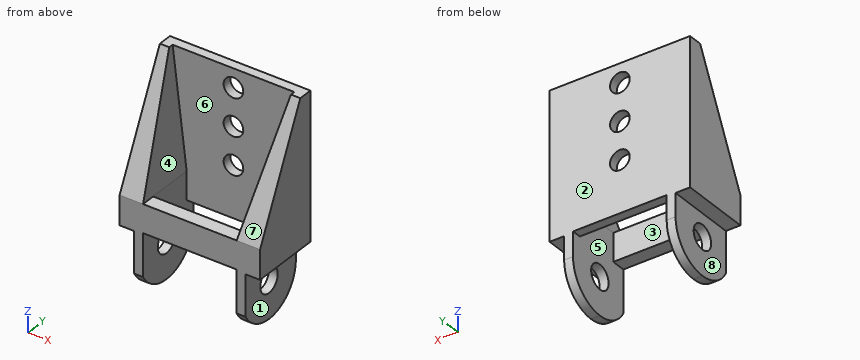
```python
from build123d import *

# Parameters (mm, degrees)
SKETCH_1_W               = 30
SKETCH_1_H               = 15
EXTRUDE_1_DEPTH          = 18
CUT_EXTRUDE_1_REACH      = 28.843
SKETCH_2_W               = 20
SKETCH_2_H               = 10
CUT_EXTRUDE_2_REACH      = 29.668
SKETCH_3_W               = 20
SKETCH_3_H               = 12
EXTRUDE_4_DEPTH          = 20
SKETCH_10_R              = 2.6
CUT_EXTRUDE_8_DEPTH      = 35.965796737
CUT_EXTRUDE_9_DEPTH      = 35.965796737
CUT_EXTRUDE_9_DEPTH_BACK = 35.965796737
SKETCH_12_W              = 1.696031958
SKETCH_12_H              = 15
SKETCH_17_W              = 3.1
SKETCH_17_H              = 15
EXTRUDE_8_DEPTH          = 0.27
EXTRUDE_9_DEPTH          = 13
CHAMFER_1_SIZE           = 25
CHAMFER_1_SIZE2          = 12
SKETCH_19_R              = 2.1
CUT_EXTRUDE_10_DEPTH     = 13
CHAMFER_2_SIZE           = 25
CHAMFER_2_SIZE_2         = 3


with BuildPart() as part:
    # 草圖1 → 填料-伸長1 (new body)
    with BuildSketch(Plane.XY):
        with Locations((2.249045701, -2.44972067)):
            Rectangle(SKETCH_1_W, SKETCH_1_H)
    extrude(amount=EXTRUDE_1_DEPTH)

    # 草圖2 → 除料-伸長1 (cut, up to next)
    with BuildSketch(Plane.XY.offset(18), mode=Mode.PRIVATE) as cut_extrude_1_sk1:
        with Locations((2.249045701, -1.94972067)):
            Rectangle(SKETCH_2_W, SKETCH_2_H)
    cut_extrude_1_tool1 = extrude(cut_extrude_1_sk1.sketch, amount=-CUT_EXTRUDE_1_REACH, mode=Mode.PRIVATE) & part.part
    add(cut_extrude_1_tool1.solids().sort_by_distance((2.249046, -1.949721, 18))[0], mode=Mode.SUBTRACT)

    # 草圖3 → 除料-伸長2 (cut, up to next)
    with BuildSketch(Plane(origin=(0, -6.94972067, 0), x_dir=(1, 0, 0), z_dir=(0, 1, 0)), mode=Mode.PRIVATE) as cut_extrude_2_sk1:
        with Locations((2.249045701, -12)):
            Rectangle(SKETCH_3_W, SKETCH_3_H)
    cut_extrude_2_tool1 = extrude(cut_extrude_2_sk1.sketch, amount=-CUT_EXTRUDE_2_REACH, mode=Mode.PRIVATE) & part.part
    add(cut_extrude_2_tool1.solids().sort_by_distance((2.249046, -6.949721, 12))[0], mode=Mode.SUBTRACT)

    # 草圖9 → 填料-伸長4 (add)
    with BuildSketch(Plane(origin=(0, 0, 0), x_dir=(-1, 0, 0), z_dir=(0, 0, -1))):
        Polygon((9.650954299, 5.05027933), (7.750954299, 5.05027933), (7.750954299, 3.05027933), (7.750954299, -6.94972067), (7.750954299, -9.94972067), (9.650954299, -9.94972067), align=None)
        Polygon((-12.249045701, 3.05027933), (-12.249045701, 5.05027933), (-14.149045701, 5.05027933), (-14.149045701, -9.94972067), (-12.249045701, -9.94972067), (-12.249045701, -6.94972067), align=None)
    extrude(amount=EXTRUDE_4_DEPTH)

    # 草圖10 → 除料-伸長8 (cut, through all)
    with BuildSketch(Plane(origin=(14.149045701, 0, 0), x_dir=(0, 0, -1), z_dir=(1, 0, 0))):
        with Locations((5.2, -2.94972067)):
            Circle(SKETCH_10_R)
    extrude(amount=-CUT_EXTRUDE_8_DEPTH, mode=Mode.SUBTRACT)

    # 草圖12 → 除料-伸長9 (cut, two sides: drawn at the far end of the back side and taken through both)
    with BuildSketch(Plane(origin=(14.149045701, 0, 0), x_dir=(0, 0, -1), z_dir=(1, 0, 0)).offset(-CUT_EXTRUDE_9_DEPTH_BACK)):
        with BuildLine():
            Line((18.303968042, 5.05027933), (5.2, 5.05027933))
            ThreePointArc((5.2, 5.05027933), (10.856854249, 2.707133579), (13.2, -2.94972067))
            ThreePointArc((13.2, -2.94972067), (12.091439137, -7.012732683), (9.072983346, -9.94972067))
            Line((9.072983346, -9.94972067), (18.303968042, -9.94972067))
            Line((18.303968042, -9.94972067), (18.303968042, 5.05027933))
        make_face()
        with Locations((19.151984021, -2.44972067)):
            Rectangle(SKETCH_12_W, SKETCH_12_H)
    extrude(amount=CUT_EXTRUDE_9_DEPTH + CUT_EXTRUDE_9_DEPTH_BACK, mode=Mode.SUBTRACT)

    # 草圖17 → 填料-伸長8 (add)
    with BuildSketch(Plane(origin=(0, 0, 0), x_dir=(-1, 0, 0), z_dir=(0, 0, -1))):
        with Locations((-15.699045701, -2.44972067)):
            Rectangle(SKETCH_17_W, SKETCH_17_H)
        with Locations((11.200954299, -2.44972067)):
            Rectangle(SKETCH_17_W, SKETCH_17_H)
    extrude(amount=EXTRUDE_8_DEPTH)

    # 草圖18 → 填料-伸長9 (add)
    with BuildSketch(Plane.XY.offset(18)):
        Polygon((-12.750954299, 5.05027933), (-12.750954299, -9.94972067), (-7.750954299, -9.94972067), (-7.750954299, 3.05027933), (12.249045701, 3.05027933), (12.249045701, -9.94972067), (17.249045701, -9.94972067), (17.249045701, 5.05027933), align=None)
    extrude(amount=EXTRUDE_9_DEPTH)

    # 導角1
    chamfer_1_edges = [part.edges().sort_by_distance(p)[0] for p in [
        (14.749045701, -9.94972067, 31),
        (-10.250954299, -9.94972067, 31),
    ]]
    chamfer_1_side = [part.faces().sort_by_distance(p)[0] for p in [
        (13.648461643, -9.94972067, -4.671491673),
    ]]
    chamfer(chamfer_1_edges, length=CHAMFER_1_SIZE, length2=CHAMFER_1_SIZE2, reference=chamfer_1_side[0])

    # 草圖19 → 除料-伸長10 (cut)
    with BuildSketch(Plane(origin=(0, 3.05027933, 0), x_dir=(-1, 0, 0), z_dir=(0, -1, 0))):
        with Locations(Location((-2.249045701, -27, 0), (0, 0, 90))):
            Circle(SKETCH_19_R)
        with Locations(Location((-2.249045701, -19, 0), (0, 0, 90))):
            Circle(SKETCH_19_R)
        with Locations(Location((-2.249045701, -11, 0), (0, 0, 90))):
            Circle(SKETCH_19_R)
    extrude(amount=-CUT_EXTRUDE_10_DEPTH, mode=Mode.SUBTRACT)

    # 導角2
    # the kernel refuses this chamfer: 25, 3 mm, written as the material it takes off along each edge
    with BuildSketch(Plane(origin=(12.249045701, 3.05027933, 31), x_dir=(-0.004583716135178889, 0, -0.9999894947180156), z_dir=(0, -1, 0)), Plane(origin=(-7.750954299, -62.93259543, 31), x_dir=(0.004583716135178923, 0, -0.9999894947180156), z_dir=(0, 1, 0))) as chamfer_2_piece_1:
        Polygon((CHAMFER_2_SIZE * 0.999989494718, CHAMFER_2_SIZE * 0.00458371613518), (-CHAMFER_2_SIZE_2 * 0.00458371613518, CHAMFER_2_SIZE_2 * 0.999989494718), (0, 0), align=None)
    extrude(amount=65.98287476, mode=Mode.SUBTRACT)


solid = part.part
```
CAD build for the part. Positions are in the model's coordinates, mm. Face numbers are marked on the shaded views. A direction names the side the tool comes from. Round coordinates to 2 decimals unless told otherwise and drop trailing zeros. Order: outer loops, then holes, each group sorted by start corner. A loop starts at its lowest first (then second) coordinate and runs counter-clockwise, first axis right, second up. Notation, with made-up numbers: (51, 55) - (60, 55) arc R29 cw to (60, 79) - close; hole circle Ø6 at (-14, 22). An arc over 180 degrees is marked (long way). Answer in a Markdown table with one row per item. Add a question column.
(1) Probe L1, parallel to X at y = -2, z = 3; L2, parallel to Y at x = 8.75, z = 4; L3, parallel to X at y = 3.85, z = 27. List the from-to ranges inside material, lowest first. Write a range as [from, to].
(2) Drop flat-ended pins along their axis: pin 1 Ø2.5 at (x, y) = (-11.5, -6) entering from -Z; pin 2 Ø8 at (x, y) = (10, -8) entering from -Z; pin 3 Ø8.5 at (y, z) = (-2.95, -5.2) entering from +X. Give the stop position or say it passes through.
(3) Band-saw the part on B-B on z = -10. List the corners of the cut face in (x, y).
(4) Band-saw the part on A-A on x = -6.75. List the corners of the cut face in (y, z), and give its area (3 significant figures).
(5) Mould opens along Y. For the marked faces 6, 7 and 8 say: +Y half, -Y half, draft (parallel to the pull), parting line (faces both ways), or undercut.
(6) Band-saw the part on D-D on x = 3. List the corners of the cut face in (y, z), and give its area (3 significant figures).
(7) 3-axis set-ups, long thin cutter, end or side, ignore diameter. For the marked faces 1, 2, 3, 4 and 5: which of +Z, -Z, +X, -X, +Y, -Y reach the whole face in a straight line?
(8) Band-saw the part on C-C on y = 0.75. List the corners of the cut face in (x, z).
Data:
| question | item | result |
|---|---|---|
| 1 | L1 | x = [-12.75, -7.75], [12.25, 17.25] |
| 1 | L2 | y = [-9.95, -6.95], [3.05, 5.05] |
| 1 | L3 | x = [-12.75, 0.15], [4.35, 17.25] |
| 2 | pin 1 | stops at z = -0.27 |
| 2 | pin 2 | stops at z = -13.01 |
| 2 | pin 3 | stops at x = 14.15 |
| 3 | outline | (-9.65, -9.35) - (-7.75, -9.35) - (-7.75, 3.45) - (-9.65, 3.45) - close; (12.25, -9.35) - (14.15, -9.35) - (14.15, 3.45) - (12.25, 3.45) - close |
| 4 | outline | (-9.95, 0) - (-6.95, 0) - (-6.95, 6) - (-9.95, 6) - close; (3.05, 0) - (5.05, 0) - (5.05, 31) - (3.05, 31) - close |
| 4 | area | 80.0 mm^2 |
| 5 | face 6 | undercut |
| 5 | face 7 | -Y half |
| 5 | face 8 | draft |
| 6 | outline | (-9.95, 0) - (-6.95, 0) - (-6.95, 6) - (-9.95, 6) - close; (3.05, 0) - (5.05, 0) - (5.05, 9.04) - (3.05, 9.04) - close; (3.05, 12.96) - (5.05, 12.96) - (5.05, 17.04) - (3.05, 17.04) - close; (3.05, 20.96) - (5.05, 20.96) - (5.05, 25.04) - (3.05, 25.04) - close; (3.05, 28.96) - (5.05, 28.96) - (5.05, 31) - (3.05, 31) - close |
| 6 | area | 56.5 mm^2 |
| 7 | face 1 | -Z, +X, +Y, -Y |
| 7 | face 2 | +Z, -Z, +X, -X, +Y |
| 7 | face 3 | +Z, -Z |
| 7 | face 4 | +Z, -Y |
| 7 | face 5 | -Z |
| 8 | outline | (-12.75, -0.27) - (-9.65, -0.27) - (-9.65, -12.29) - (-7.75, -12.29) - (-7.75, 6) - (-10.43, 28.29) - (-12.75, 28.29) - close; (12.25, -12.29) - (14.15, -12.29) - (14.15, -0.27) - (17.25, -0.27) - (17.25, 28.29) - (14.92, 28.29) - (12.25, 6) - close |
